Answer from the drawing. Dimensions are ordinates in mm from the lowest x, y and z of the part. A direction names the side the tool comes from. Give positions to 0.01 mm unless a question says otherwise; leave off trailing zeros. Order: outer loops, then holes, each group sorted by start corner. A loop starts at its lowest first (then second) coordinate and runs counter-clockwise, first axis right, second up. Notation, with made-up numbers: M -13,36.5 L 34,36.5 A18 ccw 34,66.5 Z; hole C 50,20 d7. An arc over 180 degrees is marked long. One line per item, written item: value.
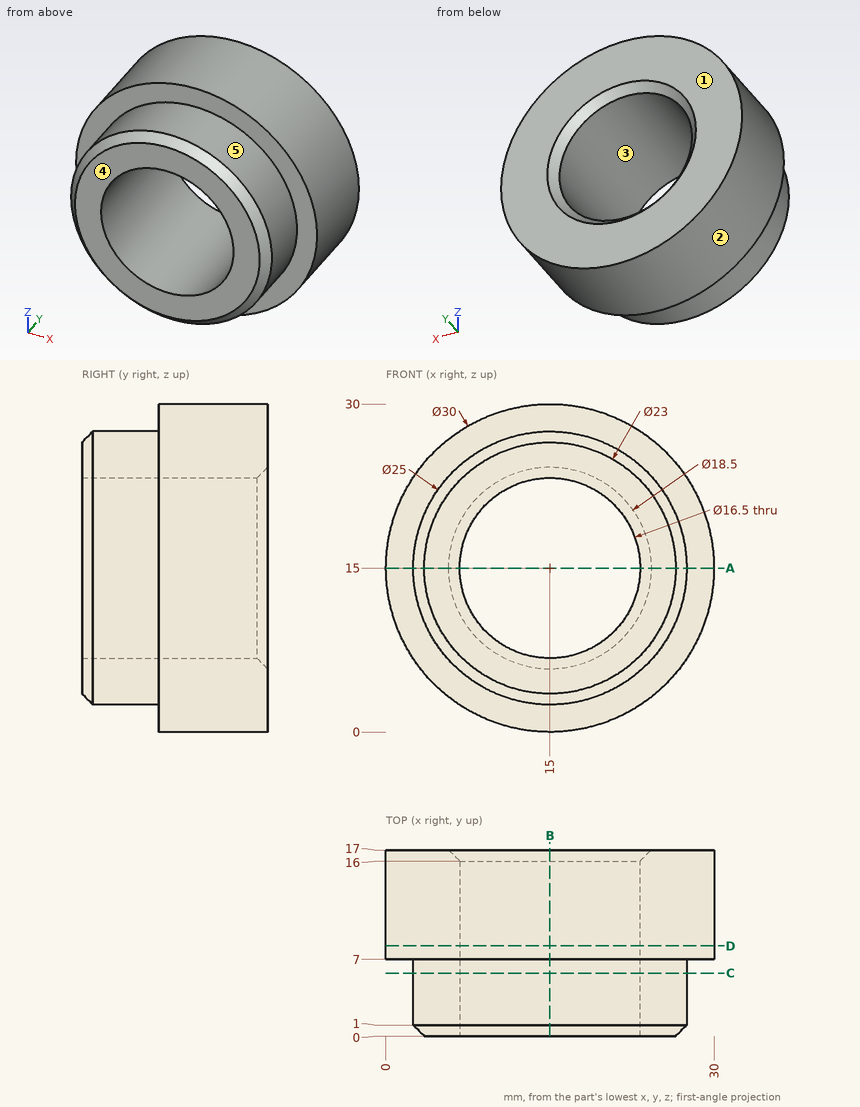
(1) Which of the six approach directions +Z, -Z, +X, -X, +Y, -Y give full straight-line access (tool end or side, diameter ignored) to the marked faces 4 and 5?
Findings:
face 4: +Z, -Z, +X, -X, -Y
face 5: -Y
(2) Given P1, Ø6, axis at x = 20, y = 7.5, coming from the +Z side; P2, Ø1, axis at x = 22.5, y = 9, coming from the -Z side; P3, Ø2, axis at y = 6.5, z = 13, coming from the +X side; P4, Ø13, axis at x = 15, z = 15, coming from the +Y side, each flat-ended and moving along its own axis, determine where each tip first touches the part or whether it passes through.
Findings:
P1: stops at z = 29.87
P2: stops at z = 1.73
P3: stops at x = 29.96
P4: passes through
(3) Section A-A, the plane z = 15 is taken. Give the vertices of the cut face in (x, y).
Findings:
outline: M 0,7 L 2.5,7 L 2.5,1 L 3.5,0 L 6.75,0 L 6.75,16 L 5.75,17 L 0,17 Z; M 23.25,0 L 26.5,0 L 27.5,1 L 27.5,7 L 30,7 L 30,17 L 24.25,17 L 23.25,16 Z
(4) Section B-B, the plane x = 15 is taken. Give the vertices of the cut face in (y, z).
Findings:
outline: M 0,3.5 L 1,2.5 L 7,2.5 L 7,0 L 17,0 L 17,5.75 L 16,6.75 L 0,6.75 Z; M 0,23.25 L 16,23.25 L 17,24.25 L 17,30 L 7,30 L 7,27.5 L 1,27.5 L 0,26.5 Z
(5) Determine the mould class of the marked faces 1, 2 and 3 for opening direction X: pulls with the +X half, pulls with the -X half, needs draft (parallel to the pull), parting line crosses it, or undercut.
Findings:
face 1: needs draft
face 2: parting line crosses it
face 3: undercut
(6) Section D-D, the plane y = 8.25 is taken. Give the vertices of the cut face in (x, z).
Findings:
outline: C 15,15 d30; hole C 15,15 d16.5
(7) Find the intervals of material crossed by probe 1 along Z at (x, y) = (15, 12.5); probe 2 along Z at (x, y) = (15, 6.5); probe 3 along Y at (x, z) = (5, 5.75), in increasing order. Write a range as from..to.
Findings:
probe 1: z = 0..6.75, 23.25..30
probe 2: z = 2.5..6.75, 23.25..27.5
probe 3: y = 7..17
(8) Section C-C, the plane y = 5.75 is taken. Give the vertices of the cut face in (x, z), then the cut area to 3 significant figures.
Findings:
outline: C 15,15 d25; hole C 15,15 d16.5
area: 277 mm^2
